Here's how the part is built. I have some questions about the finished solid (model axes, mm). A direction names the side the tool comes from. Give positions to 0.01 mm unless a question says otherwise; leave off trailing zeros. Write each loop counter-clockwise with the first axis right and the second up, starting at its lowest first coordinate (ties: lowest second). Pieces come first, ordered by that corner, then holes. Notation, with made-up numbers: M 63.25,78 L 68.25,78 A32 cw 68.25,114 Z; hole C -2.5,-6.5 d11. An arc over 180 degrees is marked long. Answer as CSV lines item,"result". Start each with the question number.
Q1. Suppose I cut it at C-C (z = -23). Write out the boundary of the cut face in (x, y), then the cut area to 3 significant figures.
Q2. Suppose I cut it at B-B (y = -11.75). Write out the boundary of the cut face in (x, z), then the cut area to 3 significant figures.
Q3. Suppose I cut it at A-A (x = 0). Write out the boundary of the cut face in (y, z).
Q4. On a 3-axis mill with a long thin cutter (end or side, diameter ignored), from which of +Z, -Z, +X, -X, +Y, -Y can I reach the whole of each face in a straight line? I mean faces 1 (the cylindrical face through (22.476, -14.511, 19.49)), 2 (the conical face through (22.1, -13.85, 19.17)), 3 (the flat face through (18.778, -10.522, 19.445)), 4 (the flat face through (-2.65, -2.54, -18.85)), 5 (the flat face through (-1, -5, 11)). Say none if no direction works.
Q5. For pin 1 (3 mm diameter, centred on y = -5.5, z = 1.5, fed in from +X); pin 2 (10.5 mm diameter, centred on x = -22.5, z = -18.5, fed in from -Y); pin 3 (6 mm diameter, centred on y = -3.5, z = -12.5, fed in from +X), each with a flat end and sliding along its axis, tell me the tip position at first contact or that it passes through.
Q6. Thinking about a two-plate mould opening in Z: for faces 6 (the flat face through (-18.75, -2.535, -3.306)), 7 (the flat face through (-12.69, -10.52, 23.87)), 8 (the flat face through (5, -5, 25)), which applies, +Z half, -Z half, draft (parallel to the pull), parting line (faces both ways), or undercut?
Q7. Suppose I cut it at D-D (x = -21). Write out the boundary of the cut face in (y, z), then the cut area to 3 significant figures.
Q8. If I drill on line 1 along Z through (x, y) = (0, -2.5); line 2 along Z through (x, y) = (0, -3.45); line 3 along X through (y, z) = (-4.75, -23), over which ranges is the centre line in solid material (lowest first)?
```python
from build123d import *

# Parameters (mm, degrees)
F0_R     = 37.5
F0_R_2   = 28.75
F0_R_3   = 10.5
F1_DEPTH = 3
F3_ANGLE = 10
F4_COUNT = 5
F5_DEPTH = 5
F6_SIZE  = 0.9
F8_DEPTH = 25


with BuildPart() as f1:
    # F0 (on Front) → F1 (new body)
    with BuildSketch(Plane.XZ):
        Circle(F0_R)
        Circle(F0_R_2, mode=Mode.SUBTRACT)
        Circle(F0_R_2)
        Circle(F0_R_3, mode=Mode.SUBTRACT)
    extrude(amount=F1_DEPTH)

    # F2 (on Top) → F3 (revolve)
    with BuildSketch(Plane.XY):
        Polygon((-25.25, -16.2), (-25.25, -3), (-28.75, -3), (-28.75, -14), (-29.75, -13.7), (-29.75, -16.2), align=None)
    revolve(axis=Axis((0, 0, 0), (0, -1, 0)), revolution_arc=F3_ANGLE)

    # F4: F1 ×5 about axis
    f4_axis = Axis((0, 0, 0), (0, -1, 0))


with BuildPart() as f1_1:
    add(f1.part)
    for i in range(1, F4_COUNT):
        add(f1.part.rotate(f4_axis, i * 360 / F4_COUNT))

    # F0 (on Front) → F5 (join)
    with BuildSketch(Plane.XZ):
        Circle(F0_R_2)
        Circle(F0_R_3, mode=Mode.SUBTRACT)
    extrude(amount=F5_DEPTH)

    # F6
    f6_edges = [f1_1.edges().sort_by_distance(p)[0] for p in [
        (-29.636792, -16.2, -2.592883),
        (-6.692294, -16.2, -28.987509),
        (25.500727, -16.2, -15.322383),
        (22.45261, -16.2, 19.517756),
        (-11.624251, -16.2, 27.385019),
    ]]
    chamfer(f6_edges, length=F6_SIZE)

    # F7 (on face) → F8 (cut)
    with BuildSketch(Plane.XZ.offset(5)):
        with BuildLine():
            ThreePointArc((-13, 0), (-11.1431749091, 6.6954949738), (-6.1031303162, 11.4783187072))
            Line((-6.1031303162, 11.4783187072), (-11.8541569603, 22.2944267197))
            ThreePointArc((-11.8541569603, 22.2944267197), (-21.6434743427, 13.0047113915), (-25.25, 0))
            Line((-25.25, 0), (-13, 0))
        make_face()
        with BuildLine():
            Line((-7.802679108, -24.0141770365), (-4.0172209269, -12.3637347118))
            ThreePointArc((-4.0172209269, -12.3637347118), (-9.8112245429, -8.5287673769), (-12.8025007892, -2.2574263097))
            Line((-12.8025007892, -2.2574263097), (-24.8663957636, -4.3846164861))
            ThreePointArc((-24.8663957636, -4.3846164861), (-19.0564169006, -16.565490482), (-7.802679108, -24.0141770365))
        make_face()
        with BuildLine():
            Line((20.427679108, -14.8415776204), (10.5172209269, -7.6412082798))
            ThreePointArc((10.5172209269, -7.6412082798), (5.0795046704, -11.9665630949), (-1.8092503125, -12.8734848936))
            Line((-1.8092503125, -12.8734848936), (-3.5141207992, -25.0042687357))
            ThreePointArc((-3.5141207992, -25.0042687357), (9.8659609944, -23.2427475497), (20.427679108, -14.8415776204))
        make_face()
        with BuildLine():
            ThreePointArc((10.5172209269, 7.6412082798), (12.3637347118, 4.0172209269), (13, 0))
            ThreePointArc((13, 0), (12.6668108422, -2.9243637065), (11.6843226019, -5.6988249083))
            Line((11.6843226019, -5.6988249083), (22.6945496691, -11.0688714564))
            ThreePointArc((22.6945496691, -11.0688714564), (24.6028441358, -5.6800141222), (25.25, 0))
            ThreePointArc((25.25, 0), (24.0141770365, 7.802679108), (20.427679108, 14.8415776204))
            Line((20.427679108, 14.8415776204), (10.5172209269, 7.6412082798))
        make_face()
        with BuildLine():
            ThreePointArc((-4.0172209269, 12.3637347118), (2.9243637065, 12.6668108422), (9.030558816, 9.3514174044))
            Line((9.030558816, 9.3514174044), (17.5401238541, 18.1633299586))
            ThreePointArc((17.5401238541, 18.1633299586), (5.6800141222, 24.6028441358), (-7.802679108, 24.0141770365))
            Line((-7.802679108, 24.0141770365), (-4.0172209269, 12.3637347118))
        make_face()
    extrude(amount=-F8_DEPTH, mode=Mode.SUBTRACT)


solid = f1_1.part
```
Resolved:
1,outline,"M -29.62,-3 L -17.25,-3 L -17.25,-5 L -10.42,-5 L -10.42,0 L -29.62,0 Z; M -7.47,-5 L -3.23,-5 L -3.23,0 L -7.47,0 Z; M 10.42,-5 L 17.25,-5 L 17.25,-3 L 29.62,-3 L 29.62,0 L 10.42,0 Z"
1,area,"164 mm^2"
2,outline,"M -28.75,0 A28.75 ccw -28.31,-4.99 L -24.87,-4.38 A25.25 cw -25.25,0 Z; M -13.5,25.38 L -11.85,22.29 A25.25 cw -7.8,24.01 L -8.88,27.34 A28.75 ccw Z; M -8.88,-27.34 A28.75 ccw -4,-28.47 L -3.51,-25 A25.25 cw -7.8,-24.01 Z; M 17.54,18.16 A25.25 cw 20.43,14.84 L 23.26,16.9 A28.75 ccw 19.97,20.68 Z; M 20.43,-14.84 L 23.26,-16.9 A28.75 ccw 25.84,-12.6 L 22.69,-11.07 A25.25 cw Z"
2,area,"82.5 mm^2"
3,outline,"M -5,-28.75 L -3,-28.75 L -3,-37.5 L 0,-37.5 L 0,-25.25 L -5,-25.25 Z; M -5,-13 L 0,-13 L 0,-10.5 L -5,-10.5 Z; M -5,10.5 L 0,10.5 L 0,13 L -5,13 Z; M -5,25.25 L 0,25.25 L 0,37.5 L -3,37.5 L -3,28.75 L -5,28.75 Z"
4,face 1,"+Z, +X, -Y"
4,face 2,"none"
4,face 3,"+Z, -X, -Y"
4,face 4,"+Y, -Y"
4,face 5,"-Y"
5,pin 1,"x = 28.75"
5,pin 2,"y = -5"
5,pin 3,"x = 36.27"
6,face 6,"undercut"
6,face 7,"-Z half"
6,face 8,"draft"
7,outline,"M -5,-19.64 L -3,-19.64 L -3,-31.07 L 0,-31.07 L 0,-14.02 L -5,-14.02 Z; M -5,-3.7 L 0,-3.7 L 0,0 L -5,0 Z; M -5,14.02 L 0,14.02 L 0,31.07 L -3,31.07 L -3,19.64 L -5,19.64 Z"
7,area,"143 mm^2"
8,line 1,"-37.5 to -25.25, -13 to -10.5, 10.5 to 13, 25.25 to 37.5"
8,line 2,"-28.75 to -25.25, -13 to -10.5, 10.5 to 13, 25.25 to 28.75"
8,line 3,"-17.25 to -10.42, -7.47 to -3.23, 10.42 to 17.25"
